Build history of the part. All positions in model axes, mm. Round coordinates to 2 decimals unless told otherwise and drop trailing zeros. Write each loop counter-clockwise with the first axis right and the second up, starting at its lowest first coordinate (ties: lowest second). Pieces come first, ordered by that corner, then holes. Notation, with made-up numbers: M 15,66 L 59,66 A16 cw 59,89 Z; hole C -35,62 d10. An arc over 180 degrees is marked long. Write item = value, one per line.
from build123d import *

# Parameters (mm, degrees)
SKETCH1_R           = 4
BOSS_EXTRUDE1_DEPTH = 2.5
FILLET1_R           = 0.5
SKETCH2_R           = 2.25
BOSS_EXTRUDE2_DEPTH = 5
SKETCH3_R           = 1.5
BOSS_EXTRUDE3_DEPTH = 5.5
CUT_EXTRUDE1_DEPTH  = 2
CUT_EXTRUDE1_DRAFT  = -6
FILLET2_R           = 0.1
LPATTERN1_COUNT     = 14
LPATTERN1_PITCH     = 0.4


with BuildPart() as part:
    # Sketch1 → Boss-Extrude1 (new body)
    with BuildSketch(Plane.XY):
        Circle(SKETCH1_R)
    extrude(amount=BOSS_EXTRUDE1_DEPTH)

    # Fillet1
    fillet1_edges = [part.edges().sort_by_distance(p)[0] for p in [
        (-4, 0, 0),
        (-4, 0, 2.5),
    ]]
    fillet(fillet1_edges, radius=FILLET1_R)

    # Sketch2 → Boss-Extrude2 (add)
    with BuildSketch(Plane(origin=(0, 0, 0), x_dir=(-1, 0, 0), z_dir=(0, 0, -1))):
        with Locations(Location((0, 0, 0), (0, 0, 180))):
            Circle(SKETCH2_R)
    extrude(amount=BOSS_EXTRUDE2_DEPTH)

    # Sketch3 → Boss-Extrude3 (add)
    with BuildSketch(Plane(origin=(0, 0, -5), x_dir=(-1, 0, 0), z_dir=(0, 0, -1))):
        Circle(SKETCH3_R)
    extrude(amount=BOSS_EXTRUDE3_DEPTH)


with BuildPart() as cut_extrude1_tool:
    # Sketch4 → Cut-Extrude1 (with draft: the straight prism first)
    with BuildSketch(Plane.XY.offset(2.5)):
        with BuildLine():
            Line((-0.4, -2), (0.4, -2))
            Line((0.4, -2), (0.4, -0.9))
            ThreePointArc((0.4, -0.9), (0.546446609, -0.546446609), (0.9, -0.4))
            Line((0.9, -0.4), (2, -0.4))
            Line((2, -0.4), (2, 0.4))
            Line((2, 0.4), (0.9, 0.4))
            ThreePointArc((0.9, 0.4), (0.546446609, 0.546446609), (0.4, 0.9))
            Line((0.4, 0.9), (0.4, 2))
            Line((0.4, 2), (-0.4, 2))
            Line((-0.4, 2), (-0.4, 0.9))
            ThreePointArc((-0.4, 0.9), (-0.546446609, 0.546446609), (-0.9, 0.4))
            Line((-0.9, 0.4), (-2, 0.4))
            Line((-2, 0.4), (-2, -0.4))
            Line((-2, -0.4), (-0.9, -0.4))
            ThreePointArc((-0.9, -0.4), (-0.546446609, -0.546446609), (-0.4, -0.9))
            Line((-0.4, -0.9), (-0.4, -2))
        make_face()
    extrude(amount=-CUT_EXTRUDE1_DEPTH)
    # Cut-Extrude1: the draft: its side faces are tilted about the plane it starts from
    cut_extrude1_sides = [cut_extrude1_tool.faces().sort_by_distance(p)[0] for p in [
        (-0.4, -1.45, 1.5),
        (0, -2, 1.5),
        (0.4, -1.45, 1.5),
        (0.546446609, -0.546446609, 1.5),
        (1.45, -0.4, 1.5),
        (2, 0, 1.5),
        (1.45, 0.4, 1.5),
        (0.546446609, 0.546446609, 1.5),
        (0.4, 1.45, 1.5),
        (0, 2, 1.5),
        (-0.4, 1.45, 1.5),
        (-0.546446609, 0.546446609, 1.5),
        (-1.45, 0.4, 1.5),
        (-2, 0, 1.5),
        (-1.45, -0.4, 1.5),
        (-0.546446609, -0.546446609, 1.5),
    ]]
    draft(cut_extrude1_sides, Plane.XY.offset(2.5), CUT_EXTRUDE1_DRAFT)


with BuildPart() as part_1:
    add(part.part)

    # Cut-Extrude1: cut by cut_extrude1_tool
    add(cut_extrude1_tool.part, mode=Mode.SUBTRACT)

    # Fillet2
    fillet2_edges = [part_1.edges().sort_by_distance(p)[0] for p in [
        (0.4, 1.45, 2.5),
        (0, 2, 2.5),
        (-0.4, 1.45, 2.5),
        (-0.546446609, 0.546446609, 2.5),
        (-1.45, 0.4, 2.5),
        (-2, 0, 2.5),
        (-1.45, -0.4, 2.5),
        (-0.546446609, -0.546446609, 2.5),
        (-0.4, -1.45, 2.5),
        (0, -2, 2.5),
        (0.4, -1.45, 2.5),
        (0.546446609, -0.546446609, 2.5),
        (1.45, -0.4, 2.5),
        (2, 0, 2.5),
        (1.45, 0.4, 2.5),
        (0.546446609, 0.546446609, 2.5),
    ]]
    fillet(fillet2_edges, radius=FILLET2_R)

    # Sketch5 → Cut-Revolve1 (revolve, cut)
    with BuildSketch(Plane(origin=(0, 0, 0), x_dir=(0, 0, -1), z_dir=(1, 0, 0)), mode=Mode.PRIVATE) as cut_revolve1_sk:
        Polygon((10.5, 1.2), (10.7, 1.51), (10.3, 1.51), align=None)
    cut_revolve1 = revolve(cut_revolve1_sk.sketch.rotate(Axis((0, 0, 3.290536828), (0, 0, -1)), 90), axis=Axis((0, 0, 3.290536828), (0, 0, -1)), mode=Mode.SUBTRACT)

    # LPattern1: Cut-Revolve1 ×14
    with Locations(*[(0, 0, i * LPATTERN1_PITCH) for i in range(1, LPATTERN1_COUNT)]):
        add(cut_revolve1, mode=Mode.SUBTRACT)


solid = part_1.part
1. Mould opens along X. For faces 1 (the face through (1.44, -0.29, 1.47)), 2 (the face through (-1.66, -1.52, -2.46)), 3 (the face through (-2, 0, -5)) say: pulls with the +X half, pulls with the -X half, needs draft (parallel to the pull), parting line crosses it, or undercut.
Responses:
face_1 = undercut
face_2 = parting line crosses it
face_3 = needs draft
2. Band-saw the part on A-A (z = 0.75). List the corners of the cut face in (x, y), plus the area to 3 significant figures.
Responses:
outline = C 0,0 d8; hole M -1.82,-0.22 L -0.9,-0.22 A0.68 cw -0.22,-0.9 L -0.22,-1.82 L 0.22,-1.82 L 0.22,-0.9 A0.68 cw 0.9,-0.22 L 1.82,-0.22 L 1.82,0.22 L 0.9,0.22 A0.68 cw 0.22,0.9 L 0.22,1.82 L -0.22,1.82 L -0.22,0.9 A0.68 cw -0.9,0.22 L -1.82,0.22 Z
area = 46.9 mm²
3. Probe probe 1 along Z at (x, y) = (-0.5, -2); probe 2 along Z at (x, y) = (2.5, 1.5); probe 3 along Y at (x, z) = (1.75, 1.75). List the from-to ranges inside material, lowest first.
Responses:
probe_1 = -5 to 2.5
probe_2 = 0 to 2.5
probe_3 = -3.6 to -0.32, 0.32 to 3.6
4. Flat gauge pin, fed straight in: pin 1 (1.5 mm diameter, centred on y = -2, z = -8.5, fed in from -X). Where does the tip first touch, or does it go through?
Responses:
pin_1 = -0.79
5. Band-saw the part on B-B (z = -3). List the corners of the cut face in (x, y).
Responses:
outline = C 0,0 d4.5
